Could you check a few things on this model? Use its own coordinates, in mm. Face numbers are marked on the shaded views. A direction names the side the tool comes from. Coordinates: 2 decimals unless noted, no trailing zeros. Loops run counter-clockwise (first coordinate to the right, second up) from the corner with the lowest first, then second, coordinate; pieces in that order, holes last. Notation, with made-up numbers: (86, 64.25) -> (91, 64.25) arc R28 ccw to (91, 88.25) -> close; hole circle Ø3 at (21, 8.25). An arc over 180 degrees is marked (long way). One line per question, with ' | ' between items.
from build123d import *

# Parameters (mm, degrees)
CUT_EXTRUDE1_DEPTH              = 30.025161498
CUT_EXTRUDE1_DEPTH_BACK         = 30.025161498
SKETCH2_R                       = 1.9
BOSS_EXTRUDE3_DEPTH             = 1.5
FILLET1_RADIUS                  = 0.9
FILLET1_LENGTH                  = 1.5
FILLET2_R                       = 0.25
CIRPATTERN5_COUNT               = 6
FILLET1_OF_CIRPATTERN5_2_RADIUS = 0.9
FILLET1_OF_CIRPATTERN5_2_LENGTH = 1.5
FILLET1_OF_CIRPATTERN5_3_RADIUS = 0.9
FILLET1_OF_CIRPATTERN5_3_LENGTH = 1.5
FILLET1_OF_CIRPATTERN5_4_RADIUS = 0.9
FILLET1_OF_CIRPATTERN5_4_LENGTH = 1.5
FILLET1_OF_CIRPATTERN5_5_RADIUS = 0.9
FILLET1_OF_CIRPATTERN5_5_LENGTH = 1.5
FILLET1_OF_CIRPATTERN5_6_RADIUS = 0.9
FILLET1_OF_CIRPATTERN5_6_LENGTH = 1.5
FILLET3_R                       = 0.25


with BuildPart() as part:
    # Sketch1 → Revolve1 (revolve)
    with BuildSketch(Plane(origin=(0, 0, 0), x_dir=(0, 0, -1), z_dir=(1, 0, 0))):
        Polygon((0, 8), (3, 8), (3, 6), (5, 6), (5, 3), (5.3, 0), (5.9, 0), (5.9, 7.2), (5.1, 7.2), (4.6, 8.5), (3.75, 8.5), (3.75, 14.3), (3.4, 14.3), (3.4, 20.2), (3.2, 20.2), (3.2, 24.05), (3.4, 24.288350719), (3.4, 26.311649281), (3.2, 26.55), (3.2, 27.8), (2.15, 27.8), (2.15, 18.4), (1.9, 18.4), (1.9, 11.4), (0, 11.4), align=None)
    revolve(axis=Axis((0, 0, 0), (0, 1, 0)))

    # Sketch2 → Cut-Extrude1 (cut, two sides: drawn at the far end of the back side and taken through both)
    with BuildSketch(Plane.XY.offset(-CUT_EXTRUDE1_DEPTH_BACK)):
        with Locations((0, 11.5)):
            Circle(SKETCH2_R)
    extrude(amount=CUT_EXTRUDE1_DEPTH + CUT_EXTRUDE1_DEPTH_BACK, mode=Mode.SUBTRACT)

    # Sketch6 → Boss-Extrude3 (add)
    with BuildSketch(Plane(origin=(0, 7.2, 0), x_dir=(1, 0, 0), z_dir=(0, 1, 0))):
        Polygon((-3.477462054, 6.043522717), (-3.030086713, 4.963463101), (-1.367103554, 5.652293279), (-1.814478896, 6.732352896), align=None)
    boss_extrude3 = extrude(amount=-BOSS_EXTRUDE3_DEPTH)

    # Fillet1: full round fillet: the end face becomes a half cylinder, R = half its width
    fillet1_face = Plane((-2.645970475, 6.45, -6.387937807), x_dir=(0, 1, 0), z_dir=(-0.382683432365, 0, -0.923879532511))  # on the end face: x along it, z out of the body
    fillet1_slab = fillet1_face.offset(-FILLET1_RADIUS / 2) * Box(FILLET1_LENGTH, 2 * FILLET1_RADIUS, FILLET1_RADIUS, mode=Mode.PRIVATE)  # the body's end, R deep
    fillet1_round = Plane((-2.301555386, 6.45, -5.556446228), x_dir=(-0.382683432365, 0, -0.923879532511), z_dir=(0, 1, 0)) * Cylinder(FILLET1_RADIUS, FILLET1_LENGTH, mode=Mode.PRIVATE)  # its axis R under the face
    add(fillet1_slab - fillet1_round, mode=Mode.SUBTRACT)

    # Fillet2
    fillet2_edges = [part.edges().sort_by_distance(p)[0] for p in [
        (-3.097973615, 5.7, -5.12735658),
        (-2.645970475, 5.7, -6.387937807),
        (-1.434990456, 5.7, -5.816186758),
    ]]
    fillet(fillet2_edges, radius=FILLET2_R)

    # CirPattern5: Boss-Extrude3 ×6 about axis
    cirpattern5_axis = Axis((0, 0, 0), (0, 1, 0))
    for i in range(1, CIRPATTERN5_COUNT):
        add(boss_extrude3.rotate(cirpattern5_axis, i * 360 / CIRPATTERN5_COUNT))

    # Fillet1 of CirPattern5 2: full round fillet: the end face becomes a half cylinder, R = half its width
    fillet1_of_cirpattern5_2_face = Plane((-6.855101656, 6.45, -0.902491254), x_dir=(0, 1, 0), z_dir=(-0.991444861374, 0, -0.13052619222))  # on the end face: x along it, z out of the body
    fillet1_of_cirpattern5_2_slab = fillet1_of_cirpattern5_2_face.offset(-FILLET1_OF_CIRPATTERN5_2_RADIUS / 2) * Box(FILLET1_OF_CIRPATTERN5_2_LENGTH, 2 * FILLET1_OF_CIRPATTERN5_2_RADIUS, FILLET1_OF_CIRPATTERN5_2_RADIUS, mode=Mode.PRIVATE)  # the body's end, R deep
    fillet1_of_cirpattern5_2_round = Plane((-5.962801281, 6.45, -0.785017681), x_dir=(-0.991444861374, 0, -0.13052619222), z_dir=(0, 1, 0)) * Cylinder(FILLET1_OF_CIRPATTERN5_2_RADIUS, FILLET1_OF_CIRPATTERN5_2_LENGTH, mode=Mode.PRIVATE)  # its axis R under the face
    add(fillet1_of_cirpattern5_2_slab - fillet1_of_cirpattern5_2_round, mode=Mode.SUBTRACT)

    # Fillet1 of CirPattern5 3: full round fillet: the end face becomes a half cylinder, R = half its width
    fillet1_of_cirpattern5_3_face = Plane((-4.209131181, 6.45, 5.485446553), x_dir=(0, 1, 0), z_dir=(-0.608761429009, 0, 0.793353340291))  # on the end face: x along it, z out of the body
    fillet1_of_cirpattern5_3_slab = fillet1_of_cirpattern5_3_face.offset(-FILLET1_OF_CIRPATTERN5_3_RADIUS / 2) * Box(FILLET1_OF_CIRPATTERN5_3_LENGTH, 2 * FILLET1_OF_CIRPATTERN5_3_RADIUS, FILLET1_OF_CIRPATTERN5_3_RADIUS, mode=Mode.PRIVATE)  # the body's end, R deep
    fillet1_of_cirpattern5_3_round = Plane((-3.661245895, 6.45, 4.771428547), x_dir=(-0.608761429009, 0, 0.793353340291), z_dir=(0, 1, 0)) * Cylinder(FILLET1_OF_CIRPATTERN5_3_RADIUS, FILLET1_OF_CIRPATTERN5_3_LENGTH, mode=Mode.PRIVATE)  # its axis R under the face
    add(fillet1_of_cirpattern5_3_slab - fillet1_of_cirpattern5_3_round, mode=Mode.SUBTRACT)

    # Fillet1 of CirPattern5 4: full round fillet: the end face becomes a half cylinder, R = half its width
    fillet1_of_cirpattern5_4_face = Plane((2.645970475, 6.45, 6.387937807), x_dir=(0, 1, 0), z_dir=(0.382683432365, 0, 0.923879532511))  # on the end face: x along it, z out of the body
    fillet1_of_cirpattern5_4_slab = fillet1_of_cirpattern5_4_face.offset(-FILLET1_OF_CIRPATTERN5_4_RADIUS / 2) * Box(FILLET1_OF_CIRPATTERN5_4_LENGTH, 2 * FILLET1_OF_CIRPATTERN5_4_RADIUS, FILLET1_OF_CIRPATTERN5_4_RADIUS, mode=Mode.PRIVATE)  # the body's end, R deep
    fillet1_of_cirpattern5_4_round = Plane((2.301555386, 6.45, 5.556446228), x_dir=(0.382683432365, 0, 0.923879532511), z_dir=(0, 1, 0)) * Cylinder(FILLET1_OF_CIRPATTERN5_4_RADIUS, FILLET1_OF_CIRPATTERN5_4_LENGTH, mode=Mode.PRIVATE)  # its axis R under the face
    add(fillet1_of_cirpattern5_4_slab - fillet1_of_cirpattern5_4_round, mode=Mode.SUBTRACT)

    # Fillet1 of CirPattern5 5: full round fillet: the end face becomes a half cylinder, R = half its width
    fillet1_of_cirpattern5_5_face = Plane((6.855101656, 6.45, 0.902491254), x_dir=(0, 1, 0), z_dir=(0.991444861374, 0, 0.13052619222))  # on the end face: x along it, z out of the body
    fillet1_of_cirpattern5_5_slab = fillet1_of_cirpattern5_5_face.offset(-FILLET1_OF_CIRPATTERN5_5_RADIUS / 2) * Box(FILLET1_OF_CIRPATTERN5_5_LENGTH, 2 * FILLET1_OF_CIRPATTERN5_5_RADIUS, FILLET1_OF_CIRPATTERN5_5_RADIUS, mode=Mode.PRIVATE)  # the body's end, R deep
    fillet1_of_cirpattern5_5_round = Plane((5.962801281, 6.45, 0.785017681), x_dir=(0.991444861374, 0, 0.13052619222), z_dir=(0, 1, 0)) * Cylinder(FILLET1_OF_CIRPATTERN5_5_RADIUS, FILLET1_OF_CIRPATTERN5_5_LENGTH, mode=Mode.PRIVATE)  # its axis R under the face
    add(fillet1_of_cirpattern5_5_slab - fillet1_of_cirpattern5_5_round, mode=Mode.SUBTRACT)

    # Fillet1 of CirPattern5 6: full round fillet: the end face becomes a half cylinder, R = half its width
    fillet1_of_cirpattern5_6_face = Plane((4.209131181, 6.45, -5.485446553), x_dir=(0, 1, 0), z_dir=(0.608761429009, 0, -0.793353340291))  # on the end face: x along it, z out of the body
    fillet1_of_cirpattern5_6_slab = fillet1_of_cirpattern5_6_face.offset(-FILLET1_OF_CIRPATTERN5_6_RADIUS / 2) * Box(FILLET1_OF_CIRPATTERN5_6_LENGTH, 2 * FILLET1_OF_CIRPATTERN5_6_RADIUS, FILLET1_OF_CIRPATTERN5_6_RADIUS, mode=Mode.PRIVATE)  # the body's end, R deep
    fillet1_of_cirpattern5_6_round = Plane((3.661245895, 6.45, -4.771428547), x_dir=(0.608761429009, 0, -0.793353340291), z_dir=(0, 1, 0)) * Cylinder(FILLET1_OF_CIRPATTERN5_6_RADIUS, FILLET1_OF_CIRPATTERN5_6_LENGTH, mode=Mode.PRIVATE)  # its axis R under the face
    add(fillet1_of_cirpattern5_6_slab - fillet1_of_cirpattern5_6_round, mode=Mode.SUBTRACT)

    # Fillet3
    fillet3_edges = [part.edges().sort_by_distance(p)[0] for p in [
        (-5.754460714, 5.7, -1.66535519),
        (-4.319470258, 5.7, 4.150831569),
        (1.434990456, 5.7, 5.816186758),
        (5.754460714, 5.7, 1.66535519),
        (4.319470258, 5.7, -4.150831569),
        (-5.98940786, 5.7, 0.119245561),
        (-6.855101656, 5.7, -0.902491254),
        (-2.891434245, 5.7, 5.246602141),
        (-4.209131181, 5.7, 5.485446553),
        (3.097973615, 5.7, 5.12735658),
        (2.645970475, 5.7, 6.387937807),
        (5.98940786, 5.7, -0.119245561),
        (6.855101656, 5.7, 0.902491254),
        (2.891434245, 5.7, -5.246602141),
        (4.209131181, 5.7, -5.485446553),
    ]]
    fillet(fillet3_edges, radius=FILLET3_R)


solid = part.part
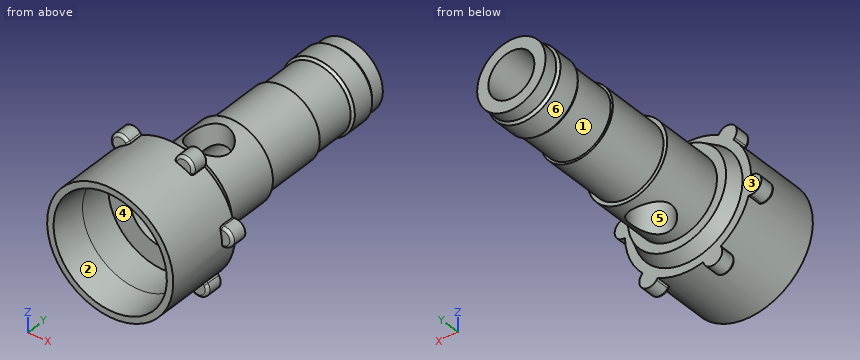
1) If we section it at B-B on y = 25: Please give me the cut outline in (x, z).
Data:
outline: circle Ø6.8 at (0, 0); hole circle Ø4.3 at (0, 0)
2) On a 3-axis mill with a long thin cutter (end or side, diameter ignored), from which of +Z, -Z, +X, -X, +Y, -Y can I reach the whole of each face in a straight line? I mean the marked faces 4, 5 and 6. Say none if no direction works.
Data:
face 4: -Y | face 5: +Z, -Z | face 6: +Y
3) We'd pull the mould along Y, two halves only. Please class the marked faces 1, 2 and 3: pulls with the +Y half, pulls with the -Y half, needs draft (parallel to the pull), parting line crosses it, or undercut.
Data:
face 1: undercut | face 2: pulls with the -Y half | face 3: pulls with the +Y half
4) I need wall thicknesses on line 1 along X through (y, z) = (22.75, 0); line 2 along Z through (x, y) = (0, 13.5); line 3 along Z through (x, y) = (0, 16.5). Which ranges of each line are inside material? Lowest first, please. Write a range as from..to.
Data:
line 1: -3.2..-2.15, 2.15..3.2 | line 2: -3.75..-1.9, 1.9..3.75 | line 3: -3.4..-1.9, 1.9..3.4
5) I'm going to push flat-ended pins straight in: pin 1 Ø3 at (y, z) = (14.5, 0.5) entering from -X; pin 2 Ø5 at (x, y) = (1.5, 12.5) entering from +Z; pin 3 Ø5 at (x, y) = (-3, 12) entering from -Z. Where does each tip first touch, or does it pass through?
Data:
pin 1: x = -3.75 | pin 2: z = 3.75 | pin 3: z = -3.66
6) If we section it at A-A on x = 0: Give the number of separate pieces and of enclosed holes in the cut face, and give its area (3 significant figures).
Data:
separate pieces: 3 | enclosed holes: 0 | area: 69.9 mm²
